from build123d import *

# Parameters (mm, degrees)
CROQUIS2_W                 = 25
CROQUIS2_H                 = 50
SALIENTE_EXTRUIR2_DEPTH    = 25
CROQUIS21_W                = 25
CROQUIS21_H                = 25
SALIENTE_EXTRUIR11_DEPTH   = 6
CROQUIS4_W                 = 39
CROQUIS4_H                 = 20
CORTAR_EXTRUIR1_DEPTH      = 9
CORTAR_EXTRUIR2_DEPTH      = 42.740268327
CORTAR_EXTRUIR2_DEPTH_BACK = 42.740268327
CROQUIS9_R                 = 8
CORTAR_EXTRUIR3_DEPTH      = 5
SALIENTE_EXTRUIR12_DEPTH   = 2
CROQUIS11_W                = 13
CROQUIS11_H                = 2
SALIENTE_EXTRUIR4_DEPTH    = 6
CROQUIS12_R                = 1.75
CORTAR_EXTRUIR4_DEPTH      = 46.345892868
CROQUIS13_W                = 13
CROQUIS13_H                = 2
SALIENTE_EXTRUIR5_DEPTH    = 6
CROQUIS14_R                = 1.75
CORTAR_EXTRUIR5_DEPTH      = 46.345892868
CROQUIS16_R                = 1.75
CORTAR_EXTRUIR6_DEPTH      = 46.345892868
CROQUIS24_R                = 1.75
CORTAR_EXTRUIR8_DEPTH      = 43.793106922
CROQUIS25_W                = 25
CROQUIS25_H                = 23
CORTAR_EXTRUIR9_DEPTH      = 6
CROQUIS28_W                = 13
CROQUIS28_H                = 8
SALIENTE_EXTRUIR13_DEPTH   = 11
REDONDEO1_R                = 4
CROQUIS29_R                = 1.75
CORTAR_EXTRUIR10_DEPTH     = 51.094909921
REDONDEO1_OF_SIMETR_A1_R   = 4
CROQUIS30_R                = 3.1
CORTAR_EXTRUIR11_DEPTH     = 3


with BuildPart() as part:
    # Croquis2 → Saliente-Extruir2 (new body)
    with BuildSketch(Plane(origin=(0, 0, 0), x_dir=(1, 0, 0), z_dir=(0, 1, 0))):
        Rectangle(CROQUIS2_W, CROQUIS2_H)
    extrude(amount=SALIENTE_EXTRUIR2_DEPTH)

    # Croquis21 → Saliente-Extruir11 (add)
    with BuildSketch(Plane.XY.offset(25)):
        with Locations((0, 12.5)):
            Rectangle(CROQUIS21_W, CROQUIS21_H)
    extrude(amount=SALIENTE_EXTRUIR11_DEPTH)

    # Croquis4 → Cortar-Extruir1 (cut, symmetric)
    with BuildSketch(Plane(origin=(0, 0, 0), x_dir=(0, 0, -1), z_dir=(1, 0, 0))):
        with Locations((-6.5, 15)):
            Rectangle(CROQUIS4_W, CROQUIS4_H)
    extrude(amount=CORTAR_EXTRUIR1_DEPTH, both=True, mode=Mode.SUBTRACT)

    # Croquis5 → Cortar-Extruir2 (cut, two sides: drawn at the far end of the back side and taken through both)
    with BuildSketch(Plane(origin=(0, 0, 0), x_dir=(0, 0, -1), z_dir=(1, 0, 0)).offset(-CORTAR_EXTRUIR2_DEPTH_BACK)):
        with BuildLine():
            ThreePointArc((2.6, 25), (-3, 30.6), (-8.6, 25))
            Line((-8.6, 25), (2.6, 25))
        make_face()
        with BuildLine():
            Line((2.6, 25), (-8.6, 25))
            ThreePointArc((-8.6, 25), (-3, 19.4), (2.6, 25))
        make_face()
    extrude(amount=CORTAR_EXTRUIR2_DEPTH + CORTAR_EXTRUIR2_DEPTH_BACK, mode=Mode.SUBTRACT)

    # Croquis9 → Cortar-Extruir3 (cut)
    with BuildSketch(Plane.XY.offset(31)):
        with Locations((0, 25)):
            Circle(CROQUIS9_R)
    extrude(amount=-CORTAR_EXTRUIR3_DEPTH, mode=Mode.SUBTRACT)

    # Croquis23 → Saliente-Extruir12 (add)
    with BuildSketch(Plane.XY.offset(31)):
        with BuildLine():
            Line((12.5, 25), (6, 25))
            ThreePointArc((6, 25), (0, 19), (-6, 25))
            Line((-6, 25), (-12.5, 25))
            Line((-12.5, 25), (-12.5, 0))
            Line((-12.5, 0), (12.5, 0))
            Line((12.5, 0), (12.5, 25))
        make_face()
    extrude(amount=SALIENTE_EXTRUIR12_DEPTH)

    # Croquis11 → Saliente-Extruir4 (add)
    with BuildSketch(Plane(origin=(12.5, 0, 0), x_dir=(0, 0, -1), z_dir=(1, 0, 0))):
        with Locations((-26.5, 24)):
            Rectangle(CROQUIS11_W, CROQUIS11_H)
    extrude(amount=SALIENTE_EXTRUIR4_DEPTH)

    # Croquis12 → Cortar-Extruir4 (cut, through all)
    with BuildSketch(Plane(origin=(0, 25, 0), x_dir=(1, 0, 0), z_dir=(0, 1, 0))):
        with Locations(Location((15.5, -23, 0), (0, 0, 270))):
            Circle(CROQUIS12_R)
        with Locations(Location((15.5, -30, 0), (0, 0, 270))):
            Circle(CROQUIS12_R)
    extrude(amount=-CORTAR_EXTRUIR4_DEPTH, mode=Mode.SUBTRACT)

    # Croquis13 → Saliente-Extruir5 (add)
    with BuildSketch(Plane.ZY.offset(12.5)):
        with Locations((26.5, 24)):
            Rectangle(CROQUIS13_W, CROQUIS13_H)
    extrude(amount=SALIENTE_EXTRUIR5_DEPTH)

    # Croquis14 → Cortar-Extruir5 (cut, through all)
    with BuildSketch(Plane(origin=(0, 25, 0), x_dir=(1, 0, 0), z_dir=(0, 1, 0))):
        with Locations(Location((-15.5, -23, 0), (0, 0, 270))):
            Circle(CROQUIS14_R)
        with Locations(Location((-15.5, -30, 0), (0, 0, 270))):
            Circle(CROQUIS14_R)
    extrude(amount=-CORTAR_EXTRUIR5_DEPTH, mode=Mode.SUBTRACT)

    # Croquis16 → Cortar-Extruir6 (cut, through all)
    with BuildSketch(Plane(origin=(0, 25, 0), x_dir=(1, 0, 0), z_dir=(0, 1, 0))):
        with Locations(Location((-7.5, 22, 0), (0, 0, 270))):
            Circle(CROQUIS16_R)
        with Locations(Location((7.5, 22, 0), (0, 0, 270))):
            Circle(CROQUIS16_R)
    extrude(amount=-CORTAR_EXTRUIR6_DEPTH, mode=Mode.SUBTRACT)

    # Croquis24 → Cortar-Extruir8 (cut, through all)
    with BuildSketch(Plane(origin=(0, 5, 0), x_dir=(1, 0, 0), z_dir=(0, 1, 0))):
        with Locations(Location((-5, -22, 0), (0, 0, 270))):
            Circle(CROQUIS24_R)
        with Locations(Location((-5, 9, 0), (0, 0, 270))):
            Circle(CROQUIS24_R)
        with Locations(Location((5, -22, 0), (0, 0, 270))):
            Circle(CROQUIS24_R)
        with Locations(Location((5, 9, 0), (0, 0, 270))):
            Circle(CROQUIS24_R)
    extrude(amount=-CORTAR_EXTRUIR8_DEPTH, mode=Mode.SUBTRACT)

    # Croquis25 → Cortar-Extruir9 (cut)
    with BuildSketch(Plane(origin=(0, 0, -25), x_dir=(-1, 0, 0), z_dir=(0, 0, -1))):
        with Locations((0, 11.5)):
            Rectangle(CROQUIS25_W, CROQUIS25_H)
    extrude(amount=-CORTAR_EXTRUIR9_DEPTH, mode=Mode.SUBTRACT)

    # Croquis28 → Saliente-Extruir13 (add)
    with BuildSketch(Plane(origin=(12.5, 0, 0), x_dir=(0, 0, -1), z_dir=(1, 0, 0))):
        with Locations((-3, 4)):
            Rectangle(CROQUIS28_W, CROQUIS28_H)
    saliente_extruir13 = extrude(amount=SALIENTE_EXTRUIR13_DEPTH)

    # Redondeo1
    redondeo1_edges = [part.edges().sort_by_distance(p)[0] for p in [
        (23.5, 0, 3),
        (23.5, 8, 3),
    ]]
    fillet(redondeo1_edges, radius=REDONDEO1_R - 0.0001)  # a hair under: the kernel refuses the full size

    # Croquis29 → Cortar-Extruir10 (cut, through all)
    with BuildSketch(Plane(origin=(0, 0, -3.5), x_dir=(-1, 0, 0), z_dir=(0, 0, -1))):
        with Locations(Location((-19.5, 4, 0), (0, 0, 90))):
            Circle(CROQUIS29_R)
    cortar_extruir10 = extrude(amount=-CORTAR_EXTRUIR10_DEPTH, mode=Mode.SUBTRACT)

    # Simetría1: Saliente-Extruir13, Cortar-Extruir10 across plane
    add(saliente_extruir13.mirror(Plane.ZY))
    add(cortar_extruir10.mirror(Plane.ZY), mode=Mode.SUBTRACT)

    # Redondeo1 of Simetría1
    redondeo1_of_simetr_a1_edges = [part.edges().sort_by_distance(p)[0] for p in [
        (-23.5, 0, 3),
        (-23.5, 8, 3),
    ]]
    fillet(redondeo1_of_simetr_a1_edges, radius=REDONDEO1_OF_SIMETR_A1_R - 0.0001)  # a hair under: the kernel refuses the full size

    # Croquis30 → Cortar-Extruir11 (cut)
    with BuildSketch(Plane(origin=(0, 5, 0), x_dir=(1, 0, 0), z_dir=(0, 1, 0))):
        with Locations(Location((-5, 9, 0), (0, 0, 270))):
            Circle(CROQUIS30_R)
        with Locations(Location((-5, -22, 0), (0, 0, 270))):
            Circle(CROQUIS30_R)
        with Locations(Location((5, -22, 0), (0, 0, 270))):
            Circle(CROQUIS30_R)
        with Locations(Location((5, 9, 0), (0, 0, 270))):
            Circle(CROQUIS30_R)
    extrude(amount=-CORTAR_EXTRUIR11_DEPTH, mode=Mode.SUBTRACT)


solid = part.part
Work out the finished part from the listing and answer in its coordinate system (mm). A direction names the side the tool comes from. Round coordinates to 2 decimals unless told otherwise and drop trailing zeros. Write each loop counter-clockwise with the first axis right and the second up, starting at its lowest first coordinate (ties: lowest second). Pieces come first, ordered by that corner, then holes. Notation, with made-up numbers: (80.25, 20) -> (107.25, 20) arc R23 ccw to (107.25, 52) -> close; hole circle Ø10 at (-12.75, 52.5). An arc over 180 degrees is marked (long way). Write each question's results on one line, items separated by ' | '.
Item 1: Find the intervals of material crossed by line 1 along X through (y, z) = (23.7, 23); line 2 along X through (y, z) = (24.35, -22); line 3 along X through (y, z) = (4, 0.5), in increasing order. Write a range as [from, to].
Result set:
line 1: [-18.5, -17.25], [-13.75, -9], [9, 13.75], [17.25, 18.5] | line 2: [-12.5, -9.25], [-5.75, 5.75], [9.25, 12.5] | line 3: [-23.5, -21.25], [-17.75, 17.75], [21.25, 23.5]
Item 2: The mould has two halves that part along Z. Classify faces 1 (the face through (3.114, 3.521, 19.54)), 2 (the face through (0, 23, -22)), 3 (the face through (17, 4, 9.5)): +Z half, -Z half, draft (parallel to the pull), parting line (faces both ways), or undercut.
Result set:
face 1: undercut | face 2: draft | face 3: +Z half
Item 3: Which of the six approach directions +Z, -Z, +X, -X, +Y, -Y give full straight-line access (tool end or side, diameter ignored) to faces 4 (the face through (12.5, 12, 4)), 5 (the face through (0, 13, 26)), 6 (the face through (-17, 4, -3.5))?
Result set:
face 4: +X | face 5: +Y | face 6: -Z, -X, +Y, -Y
Item 4: A cutting plane is placed at D-D, the plane z = 3. Count the separate pieces of the cut face and the enclosed holes in it, plus the area to 3 significant figures.
Result set:
separate pieces: 1 | enclosed holes: 2 | area: 369 mm^2
Item 5: A cutting plane is placed at A-A, the plane z = 30. Determine the outline of the cut face in (x, y).
Result set:
outline: (-18.5, 23) -> (-17.25, 23) -> (-17.25, 25) -> (-18.5, 25) -> close; (-13.75, 23) -> (-12.5, 23) -> (-12.5, 0) -> (12.5, 0) -> (12.5, 23) -> (13.75, 23) -> (13.75, 25) -> (8, 25) arc R8 cw to (-8, 25) -> (-13.75, 25) -> close; (17.25, 23) -> (18.5, 23) -> (18.5, 25) -> (17.25, 25) -> close
Item 6: A cutting plane is placed at C-C, the plane y = 16.25. Determine the outline of the cut face in (x, z).
Result set:
outline: (-12.5, -19) -> (12.5, -19) -> (12.5, 33) -> (-12.5, 33) -> close; hole (-9, -13) -> (9, -13) -> (9, 26) -> (-9, 26) -> close
Item 7: A cutting plane is placed at B-B, the plane x = 15.5. Determine the outline of the cut face in (y, z), plus the area to 3 significant figures.
Result set:
outline: (0, -3.5) -> (8, -3.5) -> (8, 9.5) -> (0, 9.5) -> close; (23, 20) -> (25, 20) -> (25, 21.25) -> (23, 21.25) -> close; (23, 24.75) -> (25, 24.75) -> (25, 28.25) -> (23, 28.25) -> close; (23, 31.75) -> (25, 31.75) -> (25, 33) -> (23, 33) -> close | area: 116 mm^2
Item 8: Flat-ended cylindrical pins translate along their axes: P1, Ø10, axis at x = -5, z = 22, coming from the +Y side; P2, Ø3.5, axis at x = -17, z = 5, coming from the +Y side; P3, Ø2.5, axis at x = 0.5, y = 20.5, coming from the -Z side; P4, Ø12, axis at y = 16.5, z = -11.5, coming from the +X side. Find the tip coordinate at first contact, or state that the pin passes through.
Result set:
P1: y = 25 | P2: y = 8 | P3: z = -19 | P4: x = 12.5
